Verification items for the finished model (mm, model axes). Round coordinates to 2 decimals unless told otherwise and drop trailing zeros. Loops run counter-clockwise (first coordinate to the right, second up) from the corner with the lowest first, then second, coordinate; pieces in that order, holes last.
from build123d import *

# Parameters (mm, degrees)
SKETCH1_R           = 11.90625
BOSS_EXTRUDE1_DEPTH = 25.4
FILLET3_R           = 5.08
FILLET4_R           = 5.08
SKETCH2_R           = 0.664162981
CUT_EXTRUDE1_DEPTH  = 25.4


with BuildPart() as part:
    # Sketch1 → Boss-Extrude1 (new body)
    with BuildSketch(Plane(origin=(0, 0, 0), x_dir=(1, 0, 0), z_dir=(0, 1, 0))):
        with Locations((-4.800132003, 11.466982006)):
            Circle(SKETCH1_R)
    extrude(amount=BOSS_EXTRUDE1_DEPTH)

    # Fillet3
    fillet3_edges = [part.edges().sort_by_distance(p)[0] for p in [
        (-16.706382003, 25.4, -11.466982006),
    ]]
    fillet(fillet3_edges, radius=FILLET3_R)

    # Fillet4
    fillet4_edges = [part.edges().sort_by_distance(p)[0] for p in [
        (-16.706382003, 0, -11.466982006),
    ]]
    fillet(fillet4_edges, radius=FILLET4_R)

    # Sketch2 → Cut-Extrude1 (cut)
    with BuildSketch(Plane(origin=(0, 25.4, 0), x_dir=(1, 0, 0), z_dir=(0, 1, 0))):
        with Locations((-4.833340152, 11.716043124)):
            Circle(SKETCH2_R)
    extrude(amount=-CUT_EXTRUDE1_DEPTH, mode=Mode.SUBTRACT)


solid = part.part
1. Section check B-B (y = 21.5). Enter the section's corners in (x, z).
2. Gauge pin test, flat ends, axial feed: P1, Ø1.5, axis at x = -11, y = 8.5, coming from the +Z side; P2, Ø6, axis at y = 9.5, z = -5, coming from the -X side; P3, Ø6, axis at x = 4, y = 9, coming from the +Z side. Record the tip position at first contact, or that the pin passes through.
3. Section check A-A (y = 17.5). Enter the section's corners in (x, z), then the cut area to 3 significant figures.
4. Scan lines: L1, parallel to Z at x = -4.5, y = 5.5; L2, parallel to Y at x = -1.5, z = -19.75; L3, parallel to Y at x = -12.5, z = -13. Record each from-to range of solid material in increasing order.
5. Release check for a two-part mould opening along X. For faces 1 (the face through (-4.92, 12.878, -12.375)), 2 (the face through (-5, 25.4, -10)), 3 (the face through (0.69, 12.59, -0.9)) record: released by +X, released by -X, zero draft, split by the parting line, or undercut.
Taken from the geometry:
1. outline: circle Ø23.53 at (-4.8, -11.47); hole circle Ø1.33 at (-4.83, -11.72)
2. P1: stops at z = -0.88
2. P2: stops at x = -16.19
2. P3: stops at z = -1.07
3. outline: circle Ø23.81 at (-4.8, -11.47); hole circle Ø1.33 at (-4.83, -11.72)
3. area: 444 mm2
4. L1: z = -23.37 to -12.29, -11.14 to 0.44
4. L2: y = 0.45 to 24.95
4. L3: y = 0.1 to 25.3
5. face 1: undercut
5. face 2: zero draft
5. face 3: split by the parting line
